Autodesk Inventor part; units mm, degrees
ref_plane "YZ Plane" through (0, 0, 0) normal (1, 0, 0) x (0, 1, 0)
ref_plane "XZ Plane" through (0, 0, 0) normal (0, 1, 0) x (-1, 0, 0)
ref_plane "XY Plane" through (0, 0, 0) normal (0, 0, 1) x (1, 0, 0)
sketch "Sketch1" plane through (0, 0, 0) normal (1, 0, 0) x (0, 1, 0)
  circle A0 centre (0, 0) radius 84.15
  dimension "d0" = 168.3
extrude "Extrude1" add sketch "Sketch1" along normal blind 286
sketch "Sketch2" plane through (0, 0, 0) normal (0, 0, 1) x (1, 0, 0)
  line L0 (0, 84.15) -> (0, -84.15)
  line L1 (286, 84.15) -> (286, -84.15)
  line L2 (0, 0) -> (286, 0) construction
  circle A0 centre (143, 0) radius 84.15
  dimension "d3" = 168.3
extrude "Extrude2" add sketch "Sketch2" along normal blind 143
sketch "Sketch3" plane through (0, 0, 0) normal (-1, 0, 0) x (0, 0, 1)
  circle A0 centre (0, 0) radius 84.15
  circle A1 centre (0, 0) radius 81.55
  dimension "d6" = 163.1
extrude "Extrude3" cut sketch "Sketch3" against normal through all contours A1
sketch "Sketch4" plane through (143, 0, 143) normal (0, 0, 1) x (1, 0, 0)
  circle A0 centre (0, 0) radius 84.15
  circle A1 centre (0, 0) radius 81.55
  dimension "d9" = 163.1
extrude "Extrude4" cut sketch "Sketch4" against normal up to next contours A1
equation "\"d0\" = d"
equation "\"d1\" = 2 * a"
equation "\"d3\" = d"
equation "\"d4\" = a"
equation "\"d6\" = d - 2 * s1"
equation "\"d7\" = a"
equation "\"d9\" = d - 2 * s1"
equation "\"d10\" = a"
equation "\"d\" = 168.3"
equation "\"s1\" = 2.6"
equation "\"a\" = 143"
equation "\"Size_Designation\" = 1.2345"
properties part number "DIN 2615-1 Tee 168.3 x 2.6 S" material "Steel"
Geometry check sheet. Reference: the model listing, model coordinates, mm. A direction names the side the tool comes from. Round coordinates to 2 decimals unless told otherwise and drop trailing zeros. Order: outer loops, then holes, each group sorted by start corner. A loop starts at its lowest first (then second) coordinate and runs counter-clockwise, first axis right, second up. Notation, with made-up numbers: M -20.75,10.5 L 30.25,10.5 A10 cw 30.25,20.5 Z; hole C 82.5,-35.5 d6. An arc over 180 degrees is marked long. Write each question's results on one line, items separated by ' | '. Start each with the question number.
1. Go/stop test with flat-tipped pins: P1, Ø5, axis at x = 210, y = 45.5, coming from the -Z side; P2, Ø1, axis at x = 31, y = -24.5, coming from the +Z side; P3, Ø10, axis at y = 31.5, z = 101, coming from the -X side. Record where each tip stops, or that it passes through.
2. Material ranges on L1, parallel to X at y = 0, z = 89; L2, parallel to X at y = 0, z = 82; L3, parallel to Z at x = 262, y = 1.5, recorded low to high. Write a range as from..to.
3. Cross-section at B-B on z = -61. Record the boundary of the cut face in (x, y).
4. Draft check along Y on faces 3 (the face through (58.93, -3.7, 102.28)), 4 (the face through (286, -69, 44)), 5 (the face through (141, 3.59, -81.47)), 6 (the face through (125.32, -79.61, 88.39)). Enter one of: pulls with the +Y half, pulls with the -Y half, needs draft (parallel to the pull), parting line crosses it, or undercut.
5. Set-up check for faces 1 (the face through (140.998, -10.955, -83.434)), 2 (the face through (74, 44, 143)): record each of +Z, -Z, +X, -X, +Y, -Y from which the full face is reachable in a straight line by a thin tool's end or side.
6. Cross-section at D-D on y = -40. Record the boundary of the cut face in (x, z), plus the area to 3 significant figures.
7. Cross-section at C-C on x = 143. Record the boundary of the cut face in (y, z), plus the area to 3 significant figures.
8. Cross-section at A-A on y = -17.5. Record the boundary of the cut face in (x, z), plus the area to 3 significant figures.
Resolved:
1) P1: z = -72.33 | P2: z = 80.65 | P3: x = 63.13
2) L1: 58.85..61.45, 224.55..227.15 | L2: 0..61.45, 224.55..286 | L3: -84.14..-81.54, 81.54..84.14
3) outline: M 0,-57.97 L 286,-57.97 L 286,-54.12 L 0,-54.12 Z; M 0,54.12 L 286,54.12 L 286,57.97 L 0,57.97 Z
4) face 3: parting line crosses it | face 4: needs draft | face 5: undercut | face 6: undercut
5) face 1: none | face 2: +Z, +X, -X, +Y, -Y
6) outline: M 0,-74.04 L 286,-74.04 L 286,-71.07 L 0,-71.07 Z; M 0,71.07 L 71.93,71.07 L 71.93,143 L 68.96,143 L 68.96,74.04 L 0,74.04 Z; M 214.07,71.07 L 286,71.07 L 286,74.04 L 217.04,74.04 L 217.04,143 L 214.07,143 Z | area: 1,690 mm2
7) outline: M -84.15,0 A84.15 ccw 84.15,0 L 84.15,143 L 81.55,143 L 81.55,0 A81.55 cw -81.55,0 L -81.55,143 L -84.15,143 Z | area: 1,420 mm2
8) outline: M 0,-82.31 L 286,-82.31 L 286,-79.65 L 0,-79.65 Z; M 0,79.65 L 63.35,79.65 L 63.35,143 L 60.69,143 L 60.69,82.31 L 0,82.31 Z; M 222.65,79.65 L 286,79.65 L 286,82.31 L 225.31,82.31 L 225.31,143 L 222.65,143 Z | area: 1,420 mm2
